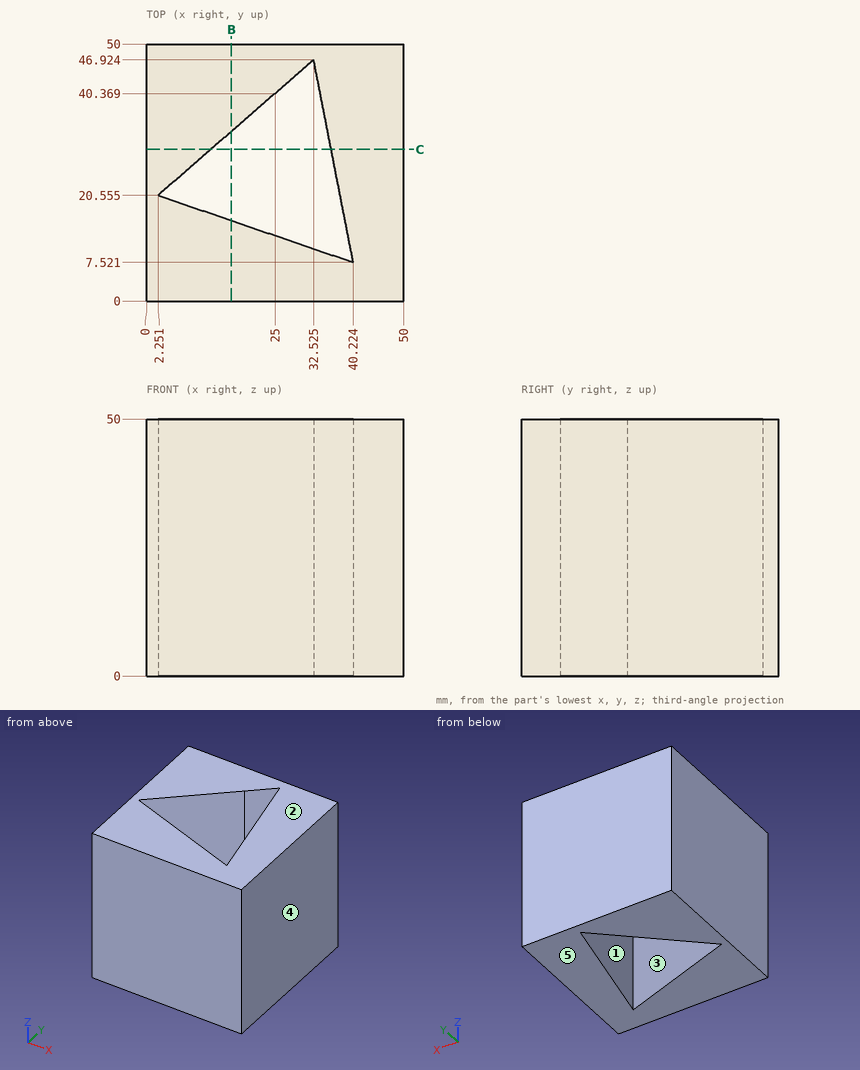
Input: dimensioned drawing with shaded views. Units: mm. Origin: part minimum x, y, z. A direction names the side the tool comes from. Round coordinates to 2 decimals unless told otherwise and drop trailing zeros. Order: outer loops, then holes, each group sorted by start corner. A loop starts at its lowest first (then second) coordinate and runs counter-clockwise, first axis right, second up. Notation, with made-up numbers: M 13,28.5 L 41,28.5 A10 ccw 41,33.5 Z; hole C 59.5,89.25 d10. An arc over 180 degrees is marked long. Use one line per item in the form item = value. Start each with the question number.
Q1. Pin query (flat end, axial travel): pin 1 Ø3 at (x, z) = (25, 41) entering from -Y. Return the tip coordinate at first contact, or that it passes through.
Q2. Mould query, pull axis X, two halves, no side actions, for the marked faces 3, 4 and 5. Classes: +X half, -X half, draft (parallel to the pull), parting line (faces both ways), or undercut.
Q3. Access query for the marked faces 1 and 2. Directions: +Z, -Z, +X, -X, +Y, -Y. A direction counts if a zero-diameter tool reaches every point of the face in a straight line with its end or side. Return the directions, or none.
Q4. Cut plane B-B (x = 16.5). Return loops of the section in (y, z) (1 decimal).
Q5. Cut plane C-C (y = 29.5). Return loops of the section in (x, z), and give its area (3 significant figures).
Q6. Material intervals for line 1 (Y direction, x = 6, z = 12); line 2 (Y direction, x = 4, z = 40) (1 decimal); line 3 (X direction, y = 32.5, z = 22) (1 decimal), sorted ascending. Write a range as [from, to].
Geometry results:
q1.pin_1 = 0
q2.face_3 = undercut
q2.face_4 = +X half
q2.face_5 = draft
q3.face_1 = +Z, -Z
q3.face_2 = +Z, +X, -X, +Y, -Y
q4.outline = M 0,0 L 15.7,0 L 15.7,50 L 0,50 Z; M 33,0 L 50,0 L 50,50 L 33,50 Z
q5.outline = M 0,0 L 12.52,0 L 12.52,50 L 0,50 Z; M 35.93,0 L 50,0 L 50,50 L 35.93,50 Z
q5.area = 1,330 mm^2
q6.line_1 = [0, 19.27], [23.82, 50]
q6.line_2 = [0, 20], [22.1, 50]
q6.line_3 = [0, 16], [35.3, 50]
